Could you check a few things on this model? Use its own coordinates, in mm. Give positions to 0.01 mm unless a question says otherwise; leave off trailing zeros. Write each loop counter-clockwise with the first axis right and the second up, starting at its lowest first coordinate (ties: lowest second). Pieces come first, ordered by that corner, then holes. Notation, with made-up numbers: (89.5, -33) - (120.5, -33) arc R16 ccw to (120.5, -24) - close; hole circle Ø1 at (-32, 51). An arc over 180 degrees is marked (long way). Answer as a JSON object with one key per item and string values. Group by question number.
```python
from build123d import *

# Parameters (mm, degrees)
PAD_DEPTH = 1


with BuildPart() as part:
    # Sketch → Pad (new body)
    with BuildSketch(Plane.XY):
        with BuildLine():
            Line((-10.160357, 55.713741), (-7.4, 55.713741))
            Line((-7.4, 55.713741), (-7.4, 7.001158))
            Line((-7.4, 7.001158), (7.4, 7.001158))
            Line((7.4, 7.001158), (7.4, 32.001158))
            Line((7.4, 32.001158), (10.160357, 32.001158))
            ThreePointArc((15.97188, 26.189635), (14.269724, 30.299002), (10.160357, 32.001158))
            Line((15.97188, 26.189635), (15.97188, 9.18934))
            Line((15.97188, 9.18934), (41.610469, -8.762993))
            ThreePointArc((42.38744, -13.169411), (42.911553, -10.805287), (41.610469, -8.762993))
            Line((42.38744, -13.169411), (37.733901, -19.815354))
            Line((37.733901, -19.815354), (17.2551, -5.475943))
            Line((17.2551, -5.475943), (4.636418, -23.497288))
            Line((4.636418, -23.497288), (43.223113, -45.775327))
            Line((43.223113, -45.775327), (41.734914, -48.352964))
            ThreePointArc((36.587732, -49.732148), (39.446961, -50.108572), (41.734914, -48.352964))
            Line((36.587732, -49.732148), (-46.367118, -1.838143))
            ThreePointArc((-49.375993, 15.369795), (-51.891139, 6.062986), (-46.367118, -1.838143))
            Line((-49.375993, 15.369795), (-18.658434, 51.765797))
            ThreePointArc((-10.160357, 55.713741), (-14.845535, 54.678573), (-18.658434, 51.765797))
        make_face()
    extrude(amount=PAD_DEPTH)


solid = part.part
```
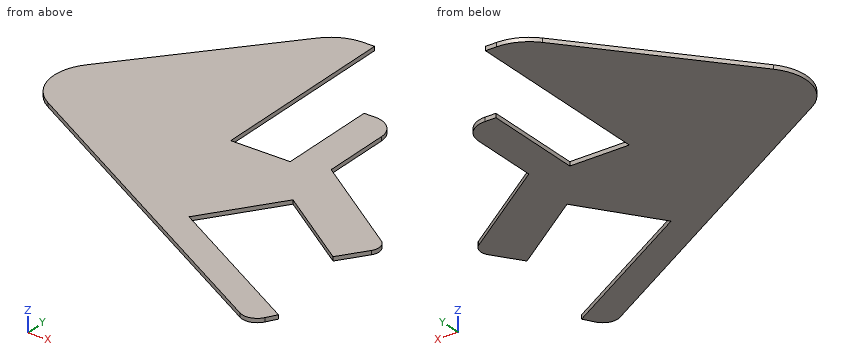
(1) I want a section at A-A, the plane y = 11.5. Please give me the cut outline in (x, z), and give its area (3 significant figures).
(2) I want a section at D-D, the plane x = -14. Please give me the cut outline in (y, z).
(3) Will these pins go through, and if not, where does the flat tip stop? P1, Ø0.5, axis at x = 8, z = 0.5, coming from the +Y side; P2, Ø0.5, axis at y = 20, z = 0.5, coming from the +X side.
(4) I want a section at B-B, the plane z = 0.45. Please give me the cut outline in (x, y).
(5) I want a section at C-C, the plane x = 6. Please give me the cut outline in (y, z).
(6) I need wall thicknesses on L1, parallel to X at y = 21.5, z = 0.5; L2, parallel to Y at x = 28, z = 0.9; L3, parallel to Y at x = 27, z = 0.1. Which ranges of each line are inside material? Lowest first, please.
Entries:
{
 "1": {"outline": "(-51.52, 0) - (-7.4, 0) - (-7.4, 1) - (-51.52, 1) - close; (7.4, 0) - (15.97, 0) - (15.97, 1) - (7.4, 1) - close", "area": "52.7 mm^2"},
 "2": {"outline": "(-20.53, 0) - (55.03, 0) - (55.03, 1) - (-20.53, 1) - close"},
 "3": {"P1": "y = 32", "P2": "x = 15.97"},
 "4": {"outline": "(-49.38, 15.37) arc R11.39 ccw to (-46.37, -1.84) - (36.59, -49.73) arc R3.77 ccw to (41.73, -48.35) - (43.22, -45.78) - (4.64, -23.5) - (17.26, -5.48) - (37.73, -19.82) - (42.39, -13.17) arc R3.16 ccw to (41.61, -8.76) - (15.97, 9.19) - (15.97, 26.19) arc R5.81 ccw to (10.16, 32) - (7.4, 32) - (7.4, 7) - (-7.4, 7) - (-7.4, 55.71) - (-10.16, 55.71) arc R11.12 ccw to (-18.66, 51.77) - close"},
 "5": {"outline": "(-32.07, 0) - (-24.28, 0) - (-24.28, 1) - (-32.07, 1) - close; (-21.55, 0) - (7, 0) - (7, 1) - (-21.55, 1) - close"},
 "6": {"L1": "-44.2 to -7.4, 7.4 to 15.97", "L2": "-44.77 to -36.99, -13 to 0.77", "L3": "-44.2 to -36.41, -12.3 to 1.47"}
}
